Part model, mm, in its own coordinate system. Face numbers are marked on the shaded views. A direction names the side the tool comes from. Round coordinates to 2 decimals unless told otherwise and drop trailing zeros. Loops run counter-clockwise (first coordinate to the right, second up) from the corner with the lowest first, then second, coordinate; pieces in that order, holes last.
(1) Cut at C-C on y = 0.25. List the corners of the cut face in (x, z).
(2) Flat gauge pins, fed straight in: pin 1 (1.5 mm diameter, centred on y = -4, z = 7, fed in from +X); pin 2 (0.5 mm diameter, centred on x = -33.5, z = 15, fed in from -Y). Where does each tip first touch, or does it go through?
(3) Probe probe 1 along Y at (x, z) = (-29.5, 18.75); probe 2 along X at (y, z) = (-3.25, 17.75); probe 3 along X at (y, z) = (5.5, 13). List the from-to ranges inside material, lowest first.
(4) Mould opens along X. For the marked faces 1, 2, 3 and 4 say: +X half, -X half, draft (parallel to the pull), parting line (faces both ways), or undercut.
(5) Cut at D-D on x = -25. List the corners of the cut face in (y, z), then the cut area to 4 significant figures.
(6) Tool access for the marked faces 5, 6, 7, 8 and 9: list every direction of +Z, -Z, +X, -X, +Y, -Y with a clear straight run to the whole face (end or side of a thin tool).
(7) Cut at B-B on x = 0. List the corners of the cut face in (y, z), then the cut area to 3 significant figures.
(8) Cut at A-A on y = 3.75. List the corners of the cut face in (x, z), then the cut area to 3 significant figures.
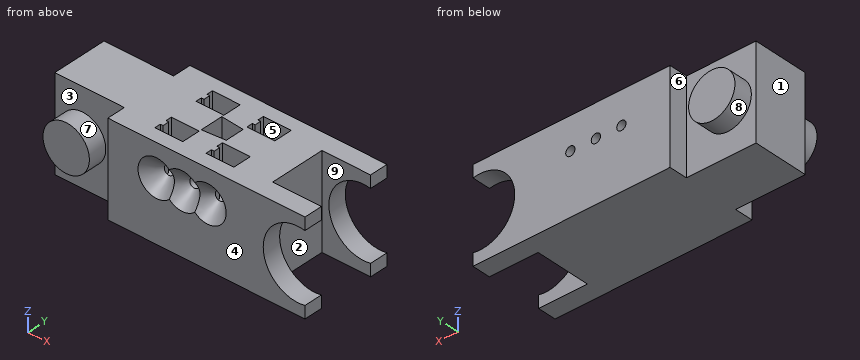
from build123d import *

# Parameters (mm, degrees)
BOSS_EXTRUDE1_DEPTH = 20
SKETCH2_R           = 5
BOSS_EXTRUDE2_DEPTH = 4
CUT_EXTRUDE1_REACH  = 64.738
SKETCH3_R           = 7.5
CUT_EXTRUDE2_DEPTH  = 10
SKETCH5_W           = 6
SKETCH5_H           = 4
CUT_EXTRUDE3_DEPTH  = 10
CUT_EXTRUDE4_REACH  = 64.738
SKETCH6_R           = 1
CHAMFER1_SIZE       = 3
SKETCH7_W           = 1.173916184
SKETCH7_H           = 1.359310186
BOSS_EXTRUDE3_DEPTH = 10


with BuildPart() as part:
    # Sketch1 → Boss-Extrude1 (new body)
    with BuildSketch(Plane.XY):
        Polygon((-41, -10), (-41, -6), (-50, -6), (-56, -6), (-56, 6), (-50, 6), (-41, 6), (-41, 10), (0, 10), (1.5, 10), (1.5, 6), (0, 6), (-9, 6), (-9, -6), (0, -6), (1.5, -6), (1.5, -10), (0, -10), align=None)
    extrude(amount=BOSS_EXTRUDE1_DEPTH)

    # Sketch2 → Boss-Extrude2 (add)
    with BuildSketch(Plane.XZ.offset(6)):
        with Locations(Location((-50, 10, 0), (0, 0, 180))):
            Circle(SKETCH2_R)
    boss_extrude2 = extrude(amount=BOSS_EXTRUDE2_DEPTH)

    # Cut-Extrude1: up to this face of the body (flat: up to its plane)
    cut_extrude1_end = Plane(part.part.faces().sort_by_distance((-19.75, 10, 10))[0])
    # Sketch3 → Cut-Extrude1 (cut, up to the picked face)
    with BuildSketch(Plane.XZ.offset(10), mode=Mode.PRIVATE) as cut_extrude1_sk1:
        with Locations((0, 10)):
            Circle(SKETCH3_R)
    cut_extrude1_tool1 = split(extrude(cut_extrude1_sk1.sketch, amount=-CUT_EXTRUDE1_REACH, mode=Mode.PRIVATE), bisect_by=cut_extrude1_end, keep=Keep.BOTH, mode=Mode.PRIVATE)
    add(cut_extrude1_tool1.solids().sort_by(Axis((0, -10, 10), (0, 1, 0)))[0], mode=Mode.SUBTRACT)

    # Mirror1: Boss-Extrude2 across plane
    add(boss_extrude2.mirror(Plane.ZX))

    # Sketch4 → Cut-Extrude2 (cut)
    with BuildSketch(Plane.XY.offset(20)):
        Polygon((-27.5, 2.5), (-22.5, 2.062556682), (-22.5, -2.062556682), (-27.5, -2.5), align=None)
    extrude(amount=-CUT_EXTRUDE2_DEPTH, mode=Mode.SUBTRACT)

    # Sketch5 → Cut-Extrude3 (cut)
    with BuildSketch(Plane.XY.offset(20)):
        with Locations((-30.5, 5)):
            Rectangle(SKETCH5_W, SKETCH5_H)
        with Locations((-19.5, 5)):
            Rectangle(SKETCH5_W, SKETCH5_H)
        with Locations((-19.5, -5)):
            Rectangle(SKETCH5_W, SKETCH5_H)
        with Locations((-30.5, -5)):
            Rectangle(SKETCH5_W, SKETCH5_H)
    extrude(amount=-CUT_EXTRUDE3_DEPTH, mode=Mode.SUBTRACT)

    # Cut-Extrude4: up to this face of the body (flat: up to its plane)
    cut_extrude4_end = Plane(part.part.faces().sort_by_distance((-22.349651974, 10, 10))[0])
    # Sketch6 → Cut-Extrude4 (cut, up to the picked face)
    with BuildSketch(Plane.XZ.offset(10), mode=Mode.PRIVATE) as cut_extrude4_sk1:
        with Locations((-30.5, 13)):
            Circle(SKETCH6_R)
    cut_extrude4_tool1 = split(extrude(cut_extrude4_sk1.sketch, amount=-CUT_EXTRUDE4_REACH, mode=Mode.PRIVATE), bisect_by=cut_extrude4_end, keep=Keep.BOTH, mode=Mode.PRIVATE)
    # Sketch6 → Cut-Extrude4 (cut, up to the picked face)
    with BuildSketch(Plane.XZ.offset(10), mode=Mode.PRIVATE) as cut_extrude4_sk2:
        with Locations((-25, 13)):
            Circle(SKETCH6_R)
    cut_extrude4_tool2 = split(extrude(cut_extrude4_sk2.sketch, amount=-CUT_EXTRUDE4_REACH, mode=Mode.PRIVATE), bisect_by=cut_extrude4_end, keep=Keep.BOTH, mode=Mode.PRIVATE)
    # Sketch6 → Cut-Extrude4 (cut, up to the picked face)
    with BuildSketch(Plane.XZ.offset(10), mode=Mode.PRIVATE) as cut_extrude4_sk3:
        with Locations(Location((-19.5, 13, 0), (0, 0, 270))):
            Circle(SKETCH6_R)
    cut_extrude4_tool3 = split(extrude(cut_extrude4_sk3.sketch, amount=-CUT_EXTRUDE4_REACH, mode=Mode.PRIVATE), bisect_by=cut_extrude4_end, keep=Keep.BOTH, mode=Mode.PRIVATE)
    add(cut_extrude4_tool1.solids().sort_by(Axis((-30.5, -10, 13), (0, 1, 0)))[0], mode=Mode.SUBTRACT)
    add(cut_extrude4_tool2.solids().sort_by(Axis((-25, -10, 13), (0, 1, 0)))[0], mode=Mode.SUBTRACT)
    add(cut_extrude4_tool3.solids().sort_by(Axis((-19.5, -10, 13), (0, 1, 0)))[0], mode=Mode.SUBTRACT)

    # Chamfer1
    # the kernel refuses this chamfer: 3 mm, written as the material it takes off along each edge
    with BuildSketch(Plane(origin=(-30.5, -10, 13), x_dir=(1, 0, 0), z_dir=(0, 0, -1))) as chamfer1_piece_1:
        Polygon((1 + CHAMFER1_SIZE, 0), (1, -CHAMFER1_SIZE), (1, 0), align=None)
    revolve(axis=Axis((-30.5, -10, 13), (0, -1, 0)), mode=Mode.SUBTRACT)
    with BuildSketch(Plane(origin=(-25, -10, 13), x_dir=(1, 0, 0), z_dir=(0, 0, -1))) as chamfer1_piece_2:
        Polygon((1 + CHAMFER1_SIZE, 0), (1, -CHAMFER1_SIZE), (1, 0), align=None)
    revolve(axis=Axis((-25, -10, 13), (0, -1, 0)), mode=Mode.SUBTRACT)
    with BuildSketch(Plane(origin=(-19.5, -10, 13), x_dir=(0, 0, -1), z_dir=(-1, 0, 0))) as chamfer1_piece_3:
        Polygon((1 + CHAMFER1_SIZE, 0), (1, -CHAMFER1_SIZE), (1, 0), align=None)
    revolve(axis=Axis((-19.5, -10, 13), (0, -1, 0)), mode=Mode.SUBTRACT)

    # Sketch7 → Boss-Extrude3 (add)
    with BuildSketch(Plane.XY.offset(20)):
        with Locations((-22.5, -5)):
            Rectangle(SKETCH7_W, SKETCH7_H)
        with Locations((-33.5, -5)):
            Rectangle(SKETCH7_W, SKETCH7_H)
        with Locations((-33.5, 5)):
            Rectangle(SKETCH7_W, SKETCH7_H)
        with Locations((-22.5, 5)):
            Rectangle(SKETCH7_W, SKETCH7_H)
    extrude(amount=-BOSS_EXTRUDE3_DEPTH)


solid = part.part
Final values:
1. outline: (-56, 0) - (-9, 0) - (-9, 20) - (-22.5, 20) - (-22.5, 10) - (-27.5, 10) - (-27.5, 20) - (-56, 20) - close; hole circle Ø2 at (-30.5, 13); hole circle Ø2 at (-19.5, 13)
2. pin 1: stops at x = -9
2. pin 2: stops at y = -9.86
3. probe 1: y = -10 to -7, -3 to 3, 7 to 10
3. probe 2: x = -56 to -33.5, -27.5 to -22.5, -16.5 to -9
3. probe 3: x = -56 to -32.91, -27.5 to -26, -24 to -21.91, -16.5 to -9
4. face 1: -X half
4. face 2: +X half
4. face 3: undercut
4. face 4: draft
5. outline: (-10, 0) - (10, 0) - (10, 12) - (2.28, 12) - (2.28, 10) - (-2.28, 10) - (-2.28, 12) - (-7, 12) - (-10, 9) - close; (-10, 17) - (-7, 14) - (-2.28, 14) - (-2.28, 20) - (-10, 20) - close; (2.28, 14) - (10, 14) - (10, 20) - (2.28, 20) - close
5. area: 314.5 mm2
6. face 5: +Z
6. face 6: +Z, -Z, +Y
6. face 7: -Y
6. face 8: +Y
6. face 9: +Z, -Z, +X
7. outline: (-10, 0) - (-6, 0) - (-6, 2.5) - (-10, 2.5) - close; (-10, 17.5) - (-6, 17.5) - (-6, 20) - (-10, 20) - close; (6, 0) - (10, 0) - (10, 2.5) - (6, 2.5) - close; (6, 17.5) - (10, 17.5) - (10, 20) - (6, 20) - close
7. area: 40.0 mm2
8. outline: (-56, 0) - (-9, 0) - (-9, 20) - (-16.5, 20) - (-16.5, 10) - (-22.5, 10) - (-22.5, 20) - (-27.5, 20) - (-27.5, 10) - (-33.5, 10) - (-33.5, 20) - (-56, 20) - close; hole circle Ø2 at (-25, 13)
8. area: 817 mm2
